Here's how the part is built. I have some questions about the finished solid (model axes, mm). Face numbers are marked on the shaded views. A direction names the side the tool comes from. Give positions to 0.01 mm unless a question says otherwise; leave off trailing zeros. Order: outer loops, then holes, each group sorted by start corner. A loop starts at its lowest first (then second) coordinate and runs counter-clockwise, first axis right, second up. Notation, with made-up numbers: (21.5, -16.5) - (28.5, -16.5) arc R22 cw to (28.5, -8.5) - close; hole circle Ø11 at (57, 75.25). An arc over 180 degrees is marked (long way). One line per question, with ' | ' between items.
from build123d import *

# Parameters (mm, degrees)
SKETCH1_W           = 12.8
SKETCH1_H           = 27
BOSS_EXTRUDE1_DEPTH = 6
SKETCH2_W           = 12
SKETCH2_H           = 16.6
CUT_EXTRUDE1_DEPTH  = 258.649269937
SKETCH3_W           = 0.8
SKETCH3_H           = 12
BOSS_EXTRUDE2_DEPTH = 12
SKETCH4_W           = 12
SKETCH4_H           = 9.6
CUT_EXTRUDE2_DEPTH  = 258.858772003
HOLE1_D             = 4.4
HOLE1_DEPTH         = 12.8
FILLET1_R           = 2
FILLET2_R           = 2
FILLET3_R           = 2.8
FILLET4_R           = 2.8


with BuildPart() as part:
    # Sketch1 → Boss-Extrude1 (new body)
    with BuildSketch(Plane(origin=(27.999999016, 0, 0), x_dir=(0, 0, -1), z_dir=(1, 0, 0))):
        with Locations((-19.400000091, -242.784034412)):
            Rectangle(SKETCH1_W, SKETCH1_H)
    extrude(amount=-BOSS_EXTRUDE1_DEPTH)

    # Sketch2 → Cut-Extrude1 (cut, through all)
    with BuildSketch(Plane(origin=(27.999999016, 0, 0), x_dir=(0, 0, -1), z_dir=(1, 0, 0))):
        with Locations((-19.800000091, -247.984034412)):
            Rectangle(SKETCH2_W, SKETCH2_H)
    extrude(amount=-CUT_EXTRUDE1_DEPTH, mode=Mode.SUBTRACT)

    # Sketch3 → Boss-Extrude2 (add)
    with BuildSketch(Plane.ZY.offset(-21.999999016)):
        with Locations((13.400000091, -250.284034412)):
            Rectangle(SKETCH3_W, SKETCH3_H)
    extrude(amount=BOSS_EXTRUDE2_DEPTH)

    # Sketch4 → Cut-Extrude2 (cut, through all)
    with BuildSketch(Plane.ZY.offset(-21.999999016)):
        with Locations((19.000000091, -234.084034412)):
            Rectangle(SKETCH4_W, SKETCH4_H)
    extrude(amount=-CUT_EXTRUDE2_DEPTH, mode=Mode.SUBTRACT)

    # Hole1
    with Locations(Plane(origin=(0, 0, 13.000000091), x_dir=(-1, 0, 0), z_dir=(0, 0, -1))):
        with Locations((-15.999999016, -250.284034412)):
            Hole(HOLE1_D / 2, depth=HOLE1_DEPTH)

    # Fillet1
    fillet1_edges = [part.edges().sort_by_distance(p)[0] for p in [
        (24.999999016, -239.684034412, 13.800000091),
    ]]
    fillet(fillet1_edges, radius=FILLET1_R)

    # Fillet2
    fillet2_edges = [part.edges().sort_by_distance(p)[0] for p in [
        (24.999999016, -238.884034412, 25.000000091),
    ]]
    fillet(fillet2_edges, radius=FILLET2_R)

    # Fillet3
    fillet3_edges = [part.edges().sort_by_distance(p)[0] for p in [
        (24.999999016, -239.684034412, 25.800000091),
    ]]
    fillet(fillet3_edges, radius=FILLET3_R)

    # Fillet4
    fillet4_edges = [part.edges().sort_by_distance(p)[0] for p in [
        (24.999999016, -238.884034412, 13.000000091),
    ]]
    fillet(fillet4_edges, radius=FILLET4_R)


solid = part.part
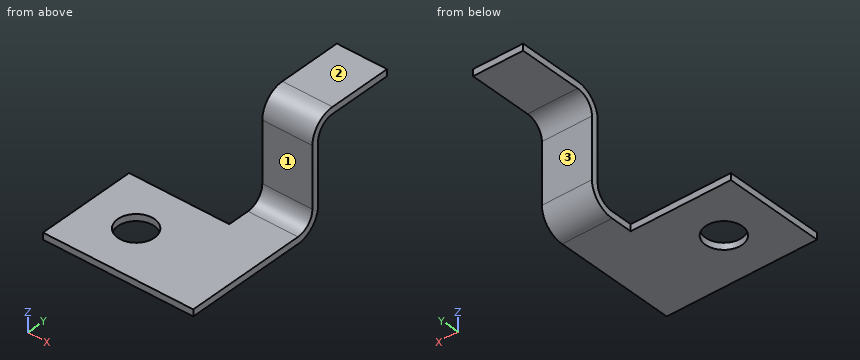
1) On a 3-axis mill with a long thin cutter (end or side, diameter ignored), from which of +Z, -Z, +X, -X, +Y, -Y can I reach the whole of each face in a straight line? I mean the marked faces 1, 2 and 3. Say none if no direction works.
Model answer:
face 1: +Z, +X, -X, -Y | face 2: +Z, +X, -X, +Y, -Y | face 3: -Z, +X, -X, +Y
2) Please list where these lines run through material, in increasing order: L1, parallel to Y at x = 16, z = 13.5; L2, parallel to Y at x = 24.5, z = 17.75; L3, parallel to Z at x = 26, y = -231.5.
Model answer:
L1: y = -256.28 to -252.48, -248.08 to -244.28 | L2: y = -239.68 to -238.88 | L3: z = 25 to 25.8
3) I want a section at D-D (z = 18). List the corners of the cut face in (x, y) for me, plus the area to 3 significant figures.
Model answer:
outline: (22, -239.68) - (28, -239.68) - (28, -238.88) - (22, -238.88) - close | area: 4.80 mm2
4) I'm going to push flat-ended pins straight in: P1, Ø4, axis at x = 12, y = -240.5, coming from the +Z side; P2, Ø4.5, axis at x = 17.5, y = -246.5, coming from the +Z side; P3, Ø5, axis at x = 25.5, y = -233, coming from the -Z side; P4, Ø3, axis at x = 25, z = 19.5, coming from the -Y side. Where does each tip first touch, or does it pass through?
Model answer:
P1: passes through | P2: stops at z = 13.8 | P3: stops at z = 25 | P4: stops at y = -239.68
5) I want a section at C-C (y = -251.75). List the corners of the cut face in (x, z) for me, plus the area to 3 significant figures.
Model answer:
outline: (10, 13) - (14.36, 13) - (14.36, 13.8) - (10, 13.8) - close; (17.64, 13) - (28, 13) - (28, 13.8) - (17.64, 13.8) - close | area: 11.8 mm2
6) I want a section at A-A (x = 16). List the corners of the cut face in (y, z) for me.
Model answer:
outline: (-256.28, 13) - (-252.48, 13) - (-252.48, 13.8) - (-256.28, 13.8) - close; (-248.08, 13) - (-244.28, 13) - (-244.28, 13.8) - (-248.08, 13.8) - close
7) I want a section at B-B (x = 24.75). List the corners of the cut face in (y, z) for me.
Model answer:
outline: (-256.28, 13) - (-241.68, 13) arc R2.8 ccw to (-238.88, 15.8) - (-238.88, 23) arc R2 cw to (-236.88, 25) - (-229.28, 25) - (-229.28, 25.8) - (-236.88, 25.8) arc R2.8 ccw to (-239.68, 23) - (-239.68, 15.8) arc R2 cw to (-241.68, 13.8) - (-256.28, 13.8) - close
